from build123d import *

# Parameters (mm, degrees)
BOSS_EXTRUDE1_DEPTH = 3


with BuildPart() as part:
    # Sketch1 → Boss-Extrude1 (new body)
    with BuildSketch(Plane.XY):
        with BuildLine():
            Line((-5, -21.5), (5, -21.5))
            ThreePointArc((5, -21.5), (13.485281374, -25.014718626), (17, -33.5))
            Line((17, -33.5), (17, -61.5))
            ThreePointArc((17, -61.5), (14.071067812, -68.571067812), (7, -71.5))
            Line((7, -71.5), (0.5, -71.5))
            Line((0.5, -71.5), (-0.5, -71.5))
            Line((-0.5, -71.5), (-7, -71.5))
            ThreePointArc((-7, -71.5), (-14.071067812, -68.571067812), (-17, -61.5))
            Line((-17, -61.5), (-17, -33.5))
            ThreePointArc((-17, -33.5), (-13.485281374, -25.014718626), (-5, -21.5))
        make_face()
    extrude(amount=BOSS_EXTRUDE1_DEPTH)


solid = part.part
Model file for the job. Use its own axes, mm. Coordinates: 2 decimals unless noted, no trailing zeros. Write each loop counter-clockwise with the first axis right and the second up, starting at its lowest first coordinate (ties: lowest second). Pieces come first, ordered by that corner, then holes. Notation, with made-up numbers: (42.25, 10.25) -> (94.25, 10.25) arc R10 ccw to (94.25, 19.25) -> close; hole circle Ø7 at (80, 53). An arc over 180 degrees is marked (long way). One line per item, written item: value. Start each with the question number.
1) Slice it at B-B on x = -11.5. Write the cut outline in (y, z), then the cut area to 3 significant figures.
2) Probe probe 1 along Y at (x, z) = (5.5, 2.25); probe 2 along X at (y, z) = (-32.5, 0.55); probe 3 along Y at (x, z) = (10, 0.45). List the from-to ranges inside material, lowest first.
3) Slice it at A-A on z = 1.25. Write the cut outline in (x, y).
4) Slice it at C-C on y = -25. Write the cut outline in (x, z), then the cut area to 3 significant figures.
Answers follow:
1. outline: (-70.43, 0) -> (-23.41, 0) -> (-23.41, 3) -> (-70.43, 3) -> close
1. area: 141 mm2
2. probe 1: -71.5 to -21.51
2. probe 2: -16.96 to 16.96
2. probe 3: -71.04 to -22.59
3. outline: (-17, -61.5) arc R10 ccw to (-7, -71.5) -> (7, -71.5) arc R10 ccw to (17, -61.5) -> (17, -33.5) arc R12 ccw to (5, -21.5) -> (-5, -21.5) arc R12 ccw to (-17, -33.5) -> close
4. outline: (-13.47, 0) -> (13.47, 0) -> (13.47, 3) -> (-13.47, 3) -> close
4. area: 80.8 mm2
